Geometry check sheet. Reference: the model listing, model coordinates, mm. Round coordinates to 2 decimals unless told otherwise and drop trailing zeros. Order: outer loops, then holes, each group sorted by start corner. A loop starts at its lowest first (then second) coordinate and runs counter-clockwise, first axis right, second up. Notation, with made-up numbers: (70.25, 44) - (79.25, 44) arc R11 cw to (79.25, 59) - close; hole circle Ø1 at (37, 76). An arc over 180 degrees is marked (long way). Write each question's results on one line, items separated by ' | '.
Autodesk Inventor part; units mm, degrees
ref_plane "YZ Plane" through (0, 0, 0) normal (1, 0, 0) x (0, 1, 0)
ref_plane "XZ Plane" through (0, 0, 0) normal (0, 1, 0) x (-1, 0, 0)
ref_plane "XY Plane" through (0, 0, 0) normal (0, 0, 1) x (1, 0, 0)
sketch "Sketch1" plane through (0, 0, 0) normal (0, 0, 1) x (1, 0, 0)
  line L0 (0, -20.5) -> (1.5, -20.5)
  line L1 (1.5, -20.5) -> (1.5, 19.5)
  line L2 (2.5, 20.5) -> (0, 20.5)
  line L3 (0, 20.5) -> (0, -20.5)
  line L4 (1.5, 19.5) -> (2.5, 20)
  line L5 (2.5, 20) -> (2.5, 20.5)
  point P0 (0, 0)
  point P1 (0, 0)
  dimension "d0" = 1.5
  dimension "d1" = 41
  dimension "d2" = 2.5
  dimension "d3" = 40
  dimension "d15" = 0.5
revolve "Revolution1" add sketch "Sketch1" angle 360 about axis through (0, 20.5, 0) along (0, -1, 0)
sketch "Sketch2" plane through (0, 20.5, 0) normal (0, 1, 0) x (1, 0, 0)
  line L0 (0, 1.2) -> (-0.4, 1.2)
  circle A0 centre (0, 0) radius 1.5
  line L1 (-1.2, 0.4) -> (-1.2, 0)
  line L2 (-0.4, 1.2) -> (-0.4, 0.4)
  line L3 (-0.4, 0.4) -> (-1.2, 0.4)
  line L4 (-1.2, 0) -> (-1.2, -0.4)
  line L5 (-1.2, -0.4) -> (-0.4, -0.4)
  line L6 (-0.4, -0.4) -> (-0.4, -1.2)
  line L7 (-0.4, -1.2) -> (0, -1.2)
  line L8 (0, -1.2) -> (0.4, -1.2)
  line L9 (0.4, -1.2) -> (0.4, -0.4)
  line L10 (0.4, -0.4) -> (1.2, -0.4)
  line L11 (1.2, -0.4) -> (1.2, 0)
  line L12 (1.2, 0) -> (1.2, 0.4)
  line L13 (1.2, 0.4) -> (0.4, 0.4)
  line L14 (0.4, 0.4) -> (0.4, 1.2)
  line L15 (0.4, 1.2) -> (0, 1.2)
  line L16 (-1.2, -0.4) -> (-1.2, 0.4)
  line L17 (-0.4, 1.2) -> (0.4, 1.2)
  line L18 (1.2, -0.4) -> (1.2, 0.4)
  line L19 (0.4, -1.2) -> (-0.4, -1.2)
  point P0 (0, 0)
  dimension "d5" = 1.2
  dimension "d6" = 1.2
  dimension "d8" = 0.4
  dimension "d11" = 360
extrude "Extrusion1" cut sketch "Sketch2" against normal blind 0.5 contours L15 L14 L13 L12 L11 L10 L9 L8 L7 L6 L5 L4 L1 L3 L2 L0
thread "Thread1"
chamfer "Chamfer1" distance 0.1 angle 45 12 edges at (-0.8, 20.5, -0.4) (-0.4, 20.5, -0.8) (0, 20.5, -1.2) (0.4, 20.5, -0.8) (0.8, 20.5, -0.4) (1.2, 20.5, 0) (0.8, 20.5, 0.4) (0.4, 20.5, 0.8) (0, 20.5, 1.2) (-0.4, 20.5, 0.8) (-1.2, 20.5, 0) (-0.8, 20.5, 0.4)
properties part number "M3x40mm"
(1) Section check A-A (x = 0). Record the cut outline in (y, z).
Answers follow:
outline: (-20.5, -1.5) - (19.5, -1.5) - (20, -2.5) - (20.5, -2.5) - (20.5, -1.3) - (20.4, -1.2) - (20, -1.2) - (20, 1.2) - (20.4, 1.2) - (20.5, 1.3) - (20.5, 2.5) - (20, 2.5) - (19.5, 1.5) - (-20.5, 1.5) - close
(2) Depth check by flat-ended pin: pin 1 Ø1.5 at (x, y) = (1.5, 4) entering from -Z; pin 2 Ø1.5 at (y, z) = (-5, 1) entering from +X; pin 3 Ø0.7 at (x, z) = (-0.5, 0) entering from +Y. Enter the tip coordinate at first touch or a pass-through.
Answers follow:
pin 1: z = -1.3 | pin 2: x = 1.48 | pin 3: y = 20
(3) Draft check along Z on faces 1 (the face through (0, -20.5, 0)), 2 (the face through (0, 20, 0)), 3 (the face through (-1.5, -0.22, -0.07)). Enter one of: released by +Z, released by -Z, zero draft, split by the parting line, or undercut.
Answers follow:
face 1: zero draft | face 2: undercut | face 3: split by the parting line
(4) Material ranges on line 1 (Y direction, x = -0.2, z = 0.35); line 2 (Y direction, x = 2.1, z = 0.5); line 3 (X direction, y = -1, z = 0.75), recorded low to high.
Answers follow:
line 1: -20.5 to 20 | line 2: 19.83 to 20.5 | line 3: -1.3 to 1.3
(5) Section check C-C (y = -15). Record the cut outline in (x, z).
Answers follow:
outline: circle Ø3 at (0, 0)
(6) Section check B-B (z = 0). Record the cut outline in (x, y).
Answers follow:
outline: (-2.5, 20) - (-1.5, 19.5) - (-1.5, -20.5) - (1.5, -20.5) - (1.5, 19.5) - (2.5, 20) - (2.5, 20.5) - (1.3, 20.5) - (1.2, 20.4) - (1.2, 20) - (-1.2, 20) - (-1.2, 20.4) - (-1.3, 20.5) - (-2.5, 20.5) - close
